```python
from build123d import *

# Parameters (mm, degrees)
HIGH_SLIDER_LINK_DEPTH = 8
SKETCH_2_R             = 2.6
PIN_BORE_DEPTH         = 67.137967524
SKETCH_3_R             = 2.6
CUT_EXTRUDE_2_DEPTH    = 67.137967524


with BuildPart() as part:
    # 草图1 → High_slider_link (new body)
    with BuildSketch(Plane.XY):
        Polygon((43.733202086, 35.819954019), (45.406009546, 37.164202316), (46.437060568, 39.046281505), (46.66938698, 41.17966209), (46.067619192, 43.239556216), (44.723370895, 44.912363676), (42.841291706, 45.943414698), (40.707911121, 46.17574111), (38.648016994, 45.573973323), (10.457407454, 30.877009652), (8.784599994, 29.532761355), (7.753548972, 27.650682166), (7.52122256, 25.517301581), (8.122990348, 23.457407454), (9.467238645, 21.784599994), (11.349317834, 20.753548972), (13.482698419, 20.52122256), (15.542592546, 21.122990348), align=None)
    extrude(amount=HIGH_SLIDER_LINK_DEPTH)

    # 草图2 → Pin_bore (cut, through all)
    with BuildSketch(Plane.XY.offset(8)):
        with Locations((41.19060954, 40.696963671)):
            Circle(SKETCH_2_R)
    extrude(amount=-PIN_BORE_DEPTH, mode=Mode.SUBTRACT)

    # 草图3 → 切除-拉伸2 (cut, through all)
    with BuildSketch(Plane.XY.offset(8)):
        with Locations((13, 26)):
            Circle(SKETCH_3_R)
    extrude(amount=-CUT_EXTRUDE_2_DEPTH, mode=Mode.SUBTRACT)


solid = part.part
```
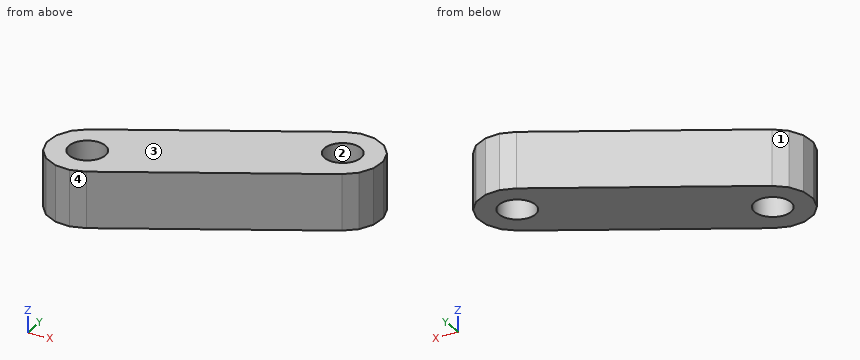
The listing builds one solid part. Answer for the finished solid, in the listing's coordinates (mm). Face numbers are marked on the shaded views. Coordinates: 2 decimals unless noted, no trailing zeros. Loops run counter-clockwise (first coordinate to the right, second up) from the corner with the lowest first, then second, coordinate; pieces in that order, holes last. Notation, with made-up numbers: (66, -33.5) -> (74, -33.5) arc R8 cw to (74, -28.5) -> close; hole circle Ø11 at (55, 32). An arc over 180 degrees is marked (long way). Return JSON: item names as keys, results as strings. Group by question number.
(1) A cutting plane is placed at D-D on y = 23. Write down the section's boundary in (x, z), and give its area (3 significant figures).
(2) A cutting plane is placed at A-A on x = 13. Write down the section's boundary in (y, z), and give its area (3 significant figures).
(3) Find the intervals of material crossed by probe 1 along X at (y, z) = (39.75, 6.25); probe 2 along X at (y, z) = (39.25, 7.5); probe 3 along Y at (x, z) = (43, 5.25), in increasing order. Write a range as from..to.
(4) A cutting plane is placed at C-C on z = 7.5. Write down the section's boundary in (x, y).
(5) Given pin 1 Ø1.5 at (y, z) = (37, 4.5) entering from +X; pin 2 Ø8 at (x, y) = (18.5, 41.5) entering from -Z; pin 3 Ø3 at (x, z) = (13, 3.5) entering from -Y, each flat-ended and moving along its own axis, determine where each tip first touches the part or whether it passes through.
(6) Determine the mould class of the marked faces 1, 2, 3 and 4 for opening direction Y: released by +Y, released by -Y, zero draft, split by the parting line, or undercut.
(7) A cutting plane is placed at B-B on y = 26. Write down the section's boundary in (x, z).
The answers:
{
 "1": {"outline": "(8.49, 0) -> (19.14, 0) -> (19.14, 8) -> (8.49, 8) -> close", "area": "85.2 mm^2"},
 "2": {"outline": "(20.57, 0) -> (23.4, 0) -> (23.4, 8) -> (20.57, 8) -> close; (28.6, 0) -> (32.2, 0) -> (32.2, 8) -> (28.6, 8) -> close", "area": "51.4 mm^2"},
 "3": {"probe 1": "x = 27.48..38.77, 43.61..46.51", "probe 2": "x = 26.52..39.03, 43.35..46.46", "probe 3": "y = 35.44..38.83, 42.56..45.86"},
 "4": {"outline": "(7.52, 25.52) -> (8.12, 23.46) -> (9.47, 21.78) -> (11.35, 20.75) -> (13.48, 20.52) -> (15.54, 21.12) -> (43.73, 35.82) -> (45.41, 37.16) -> (46.44, 39.05) -> (46.67, 41.18) -> (46.07, 43.24) -> (44.72, 44.91) -> (42.84, 45.94) -> (40.71, 46.18) -> (38.65, 45.57) -> (10.46, 30.88) -> (8.78, 29.53) -> (7.75, 27.65) -> close; hole circle Ø5.2 at (13, 26); hole circle Ø5.2 at (41.19, 40.7)"},
 "5": {"pin 1": "stops at x = 45.73", "pin 2": "passes through", "pin 3": "stops at y = 20.52"},
 "6": {"face 1": "released by +Y", "face 2": "undercut", "face 3": "zero draft", "face 4": "released by -Y"},
 "7": {"outline": "(7.57, 0) -> (10.4, 0) -> (10.4, 8) -> (7.57, 8) -> close; (15.6, 0) -> (24.9, 0) -> (24.9, 8) -> (15.6, 8) -> close"}
}
